from build123d import *

# Parameters (mm, degrees)
F0_W     = 76.2
F0_H     = 30.48
F1_DEPTH = 25.4
F2_R     = 5.08
F4_R     = 12.7
F5_DEPTH = 25.4


with BuildPart() as f1:
    # F0 (on Top) → F1 (new body)
    with BuildSketch(Plane.XY):
        Rectangle(F0_W, F0_H)
    extrude(amount=F1_DEPTH)

    # F2
    f2_edges = [f1.edges().sort_by_distance(p)[0] for p in [
        (38.1, 0, 25.4),
        (38.1, -15.24, 12.7),
        (38.1, 15.24, 12.7),
    ]]
    fillet(f2_edges, radius=F2_R)

    # F4 (on face) → F5 (join)
    with BuildSketch(Plane.XY.offset(25.4)):
        with Locations((-14.963861, 0)):
            Circle(F4_R)
    extrude(amount=F5_DEPTH)


solid = f1.part
Geometry: final body of the model. Coordinates: model frame, mm. A direction names the side the tool comes from. Coordinates: 2 decimals unless noted, no trailing zeros. Loops run counter-clockwise (first coordinate to the right, second up) from the corner with the lowest first, then second, coordinate; pieces in that order, holes last. Notation, with made-up numbers: M 68.5,53.25 L 77.5,53.25 A21 cw 77.5,77.25 Z; hole C 77,-20 d7. An arc over 180 degrees is marked long. One line per item, written item: value. Start each with the question number.
1) Material intervals for L1, parallel to Z at x = 26, y = 1; L2, parallel to X at y = 10.5, z = 19; L3, parallel to X at y = -9, z = 46, sorted ascending. Write a range as from..to.
2) Cut plane A-A (y = 0). Return loops of the section in (x, z), then the cut area to 3 significant figures.
3) Reachability of faces 1 (the cylindrical face through (36.572, -13.791, 12.878)), 2 (the cylindrical face through (-17.7, -12.4, 37.9)) from +Z, -Z, +X, -X, +Y, -Y: full face, straight path, thin tool, end or side. Return the list, or none.
4) Cut plane D-D (x = 4.5). Return loops of the section in (y, z), then the cut area to 3 significant figures.
5) Cut plane C-C (z = 48.5). Return loops of the section in (x, y), then the cut area to 3 significant figures.
6) Pin query (flat end, axial travel): P1, Ø12, axis at x = -5, z = 41, coming from the -Y side; P2, Ø2, axis at x = -10.5, y = -8, coming from the -Z side; P3, Ø4, axis at x = 10, y = 6.5, coming from the +Z side. Return the tip coordinate at first contact, or that it passes through.
7) Cut plane B-B (x = -25.5). Return loops of the section in (y, z).
Evaluation:
1. L1: 0..25.4
1. L2: -38.1..38.09
1. L3: -23.92..-6
2. outline: M -38.1,0 L 38.1,0 L 38.1,20.32 A5.08 ccw 33.02,25.4 L -2.26,25.4 L -2.26,50.8 L -27.66,50.8 L -27.66,25.4 L -38.1,25.4 Z
2. area: 2,580 mm^2
3. face 1: +Z, -Z, +X, -Y
3. face 2: +Z
4. outline: M -15.24,0 L 15.24,0 L 15.24,25.4 L -15.24,25.4 Z
4. area: 774 mm^2
5. outline: C -14.96,0 d25.4
5. area: 507 mm^2
6. P1: y = -12.07
6. P2: z = 0
6. P3: z = 25.4
7. outline: M -15.24,0 L 15.24,0 L 15.24,25.4 L 7.09,25.4 L 7.09,50.8 L -7.09,50.8 L -7.09,25.4 L -15.24,25.4 Z
